from build123d import *

# Parameters (mm, degrees)
F0_W     = 30
F0_H     = 18
F0_R     = 1.5
F1_DEPTH = 6.25
F3_DEPTH = 3.6


with BuildPart() as f1:
    # F0 (on Top) → F1 (new body)
    with BuildSketch(Plane.XY):
        Rectangle(F0_W, F0_H)
        with Locations((-12, -5.8)):
            Circle(F0_R, mode=Mode.SUBTRACT)
        with Locations((12, -5.8)):
            Circle(F0_R, mode=Mode.SUBTRACT)
        with Locations((-12, 5.8)):
            Circle(F0_R, mode=Mode.SUBTRACT)
        with Locations((12, 5.8)):
            Circle(F0_R, mode=Mode.SUBTRACT)
    extrude(amount=F1_DEPTH)

    # F2 (on face) → F3 (cut)
    with BuildSketch(Plane.XY.offset(6.25)):
        Polygon((8.5, -6.5), (8.5, 6.5), (6, 6.5), (6, 5.5), (-6, 5.5), (-6, 6.5), (-8.5, 6.5), (-8.5, -6.5), (-6, -6.5), (-6, -5.5), (6, -5.5), (6, -6.5), align=None)
    extrude(amount=-F3_DEPTH, mode=Mode.SUBTRACT)


solid = f1.part
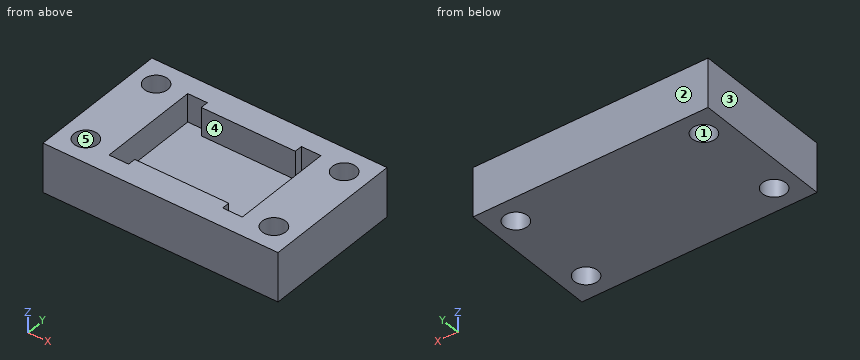
Input: part model. Units: mm. Frame: model coordinates. Face numbers are marked on the shaded views. A direction names the side the tool comes from. Round coordinates to 2 decimals unless told otherwise and drop trailing zeros. Loops run counter-clockwise (first coordinate to the right, second up) from the corner with the lowest first, then second, coordinate; pieces in that order, holes last. Notation, with made-up numbers: M -7,-10.75 L 26,-10.75 A30 cw 26,20.25 Z; hole C -19.5,88 d10. An arc over 180 degrees is marked long. Answer as CSV lines item,"result". Start each with the question number.
(1) Draft query along Y for the marked faces 1, 2 and 3. Return one class per face: released by +Y, released by -Y, zero draft, split by the parting line, or undercut.
(2) Section A-A, the plane y = -7. Output: boundary loops of the cut face in (x, z).
(3) Section C-C, the plane z = 1.5. Output: boundary loops of the cut face in (x, y), plus the area to 3 significant figures.
(4) Line query: line 1 (Y direction, x = 12, z = 4.25); line 2 (X direction, y = -0.75, z = 5.25); line 3 (X direction, y = 5.75, z = 6). Output: solid intervals per line, ascending. Write a range as [from, to].
(5) First-contact query: pin 1 (4 mm diameter, centred on x = 3, y = -1, fed in from +Z); pin 2 (1.8 mm diameter, centred on x = -12, y = -5.8, fed in from -Z); pin 3 (8 mm diameter, centred on x = 0.5, y = 3, fed in from -Z). Flat tips, straight axial feed; report the tip coordinate or a pass-through.
(6) Section B-B, the plane x = -12. Output: boundary loops of the cut face in (y, z).
(7) Reachability of the marked faces 4 and 5 from +Z, -Z, +X, -X, +Y, -Y: full face, straight path, thin tool, end or side. Return the list, or none.
(8) Section D-D, the plane y = 2.5. Output: boundary loops of the cut face in (x, z).
Values found:
1,face 1,"undercut"
1,face 2,"released by +Y"
1,face 3,"zero draft"
2,outline,"M -15,0 L -12.9,0 L -12.9,6.25 L -15,6.25 Z; M -11.1,0 L 11.1,0 L 11.1,6.25 L -11.1,6.25 Z; M 12.9,0 L 15,0 L 15,6.25 L 12.9,6.25 Z"
3,outline,"M -15,-9 L 15,-9 L 15,9 L -15,9 Z; hole C -12,-5.8 d3; hole C -12,5.8 d3; hole C 12,-5.8 d3; hole C 12,5.8 d3"
3,area,"512 mm²"
4,line 1,"y = [-9, -7.3], [-4.3, 4.3], [7.3, 9]"
4,line 2,"x = [-15, -8.5], [8.5, 15]"
4,line 3,"x = [-15, -13.5], [-10.5, -8.5], [-6, 6], [8.5, 10.5], [13.5, 15]"
5,pin 1,"stops at z = 2.65"
5,pin 2,"passes through"
5,pin 3,"stops at z = 0"
6,outline,"M -9,0 L -7.3,0 L -7.3,6.25 L -9,6.25 Z; M -4.3,0 L 4.3,0 L 4.3,6.25 L -4.3,6.25 Z; M 7.3,0 L 9,0 L 9,6.25 L 7.3,6.25 Z"
7,face 4,"+Z"
7,face 5,"+Z, -Z"
8,outline,"M -15,0 L 15,0 L 15,6.25 L 8.5,6.25 L 8.5,2.65 L -8.5,2.65 L -8.5,6.25 L -15,6.25 Z"
